Geometry check sheet. Reference: the model listing, model coordinates, mm. A direction names the side the tool comes from. Round coordinates to 2 decimals unless told otherwise and drop trailing zeros. Write each loop counter-clockwise with the first axis right and the second up, starting at its lowest first coordinate (ties: lowest second). Pieces come first, ordered by that corner, then holes.
Item 1: Draft check along Z on faces 6 (the face through (-20, -2, -20)), 7 (the face through (30, -1, 0)), 8 (the face through (32, -1, 0)), 9 (the face through (-12, -7, 5)). Enter one of: pulls with the +Z half, pulls with the -Z half, needs draft (parallel to the pull), parting line crosses it, or undercut.
Item 2: Access from +Z, -Z, +X, -X, +Y, -Y to the whole of each face (thin tool, end or side, straight path). Record for faces 1 (the face through (16.85, -22, 0)), 2 (the face through (-32, -1, 0)), 3 (the face through (22.5, -10, 0)), 4 (the face through (20, -2, -20)), 5 (the face through (-22.5, -34, 0)).
Item 3: Cross-section at A-A (z = -2). State how many separate pieces and enclosed holes the cut face has, then the cut area to 3 significant figures.
Item 4: Scan lines: probe 1 along X at (y, z) = (-25.5, 10); probe 2 along X at (y, z) = (-39, 8.5); probe 3 along Y at (x, z) = (-23, 10.5). Record each from-to range of solid material in increasing order.
Item 5: Cross-section at D-D (x = -11.5). Enter the section's corners in (y, z).
Item 6: Cross-section at B-B (y = -12.5). Enter the section's corners in (x, z).
Item 7: Depth check by flat-ended pin: P1, Ø17.5, axis at y = -30, z = -8, coming from the +X side; P2, Ø17.5, axis at y = -32, z = -4, coming from the -X side; P3, Ø4.5, axis at x = -18.5, z = -19.5, coming from the +Y side. Enter the tip coordinate at first touch or a pass-through.
Item 8: Cross-section at C-C (z = 18). Enter the section's corners in (x, y), then the cut area to 3 significant figures.
from build123d import *

# Parameters (mm, degrees)
F1_DEPTH      = 2
F2_W          = 5.6501800592
F2_H          = 10
F2_H_2        = 30
F3_DEPTH      = 40
F5_DEPTH      = 50
F7_DEPTH      = 50
F8_W          = 13.8498199408
F8_H          = 10
F9_DEPTH      = 15
F10_T4_DEPTH  = 87.150489639
F10_T10_DEPTH = 87.150489639


# Not quite as in the source:
# - a fillet or chamfer that OpenCascade refuses, or shapes differently, is made with other operations: its cross-section is extruded or revolved along the edge and cut away or added


with BuildPart() as f1:
    # F0 (on Front) → F1 (new body)
    with BuildSketch(Plane.XZ):
        with BuildLine():
            Line((32.5, 15), (-32.5, 15))
            ThreePointArc((-32.5, 15), (-34.267766953, 14.267766953), (-35, 12.5))
            Line((-35, 12.5), (-35, -12.5))
            ThreePointArc((-35, -12.5), (-34.267766953, -14.267766953), (-32.5, -15))
            Line((-32.5, -15), (32.5, -15))
            ThreePointArc((32.5, -15), (34.267766953, -14.267766953), (35, -12.5))
            Line((35, -12.5), (35, 12.5))
            ThreePointArc((35, 12.5), (34.267766953, 14.267766953), (32.5, 15))
        make_face()
        with BuildLine():
            Line((-32, -11), (-32, 11))
            ThreePointArc((-32, 11), (-31.7071067812, 11.7071067812), (-31, 12))
            ThreePointArc((-31, 12), (-30.2928932188, 11.7071067812), (-30, 11))
            Line((-30, 11), (-30, -11))
            ThreePointArc((-30, -11), (-30.2928932188, -11.7071067812), (-31, -12))
            ThreePointArc((-31, -12), (-31.7071067812, -11.7071067812), (-32, -11))
        make_face(mode=Mode.SUBTRACT)
        with BuildLine():
            Line((30, -11), (30, 11))
            ThreePointArc((30, 11), (30.2928932188, 11.7071067812), (31, 12))
            ThreePointArc((31, 12), (31.7071067812, 11.7071067812), (32, 11))
            Line((32, 11), (32, -11))
            ThreePointArc((32, -11), (31.7071067812, -11.7071067812), (31, -12))
            ThreePointArc((31, -12), (30.2928932188, -11.7071067812), (30, -11))
        make_face(mode=Mode.SUBTRACT)
    extrude(amount=F1_DEPTH)

    # F2 (on face) → F3 (join)
    with BuildSketch(Plane.XZ.offset(2)):
        with Locations((-19.6749099704, 20)):
            Rectangle(F2_W, F2_H)
        with Locations((-19.6749099704, 0)):
            Rectangle(F2_W, F2_H_2)
        with Locations((-19.6749099704, -20)):
            Rectangle(F2_W, F2_H)
        with Locations((19.6749099704, -20)):
            Rectangle(F2_W, F2_H)
        with Locations((19.6749099704, 0)):
            Rectangle(F2_W, F2_H_2)
        with Locations((19.6749099704, 20)):
            Rectangle(F2_W, F2_H)
    extrude(amount=F3_DEPTH)

    # F4 (on face) → F5 (cut, through all)
    with BuildSketch(Plane.XY.offset(25)):
        Polygon((-20.5, -17), (-22.5, -18), (-22.5, -26), (-20.5, -27), (-20.5, -26), (-20.5, -18), align=None)
    extrude(amount=-F5_DEPTH, mode=Mode.SUBTRACT)

    # F6 (on face) → F7 (cut, through all)
    with BuildSketch(Plane.XY.offset(25)):
        Polygon((22.5, -26), (22.5, -18), (20.5, -17), (20.5, -18), (20.5, -26), (20.5, -27), align=None)
    extrude(amount=-F7_DEPTH, mode=Mode.SUBTRACT)

    # F8 (on face) → F9 (join)
    with BuildSketch(Plane.XZ.offset(2)):
        with Locations((-9.9249099704, 0)):
            Rectangle(F8_W, F8_H)
        with Locations((9.9249099704, 0)):
            Rectangle(F8_W, F8_H)
    extrude(amount=F9_DEPTH)

    # F10: chamfer of 15 on 2 edges, made by hand


with BuildPart() as f10_tool2:
    # F10_s3 → F10_t4 (new body)
    with BuildSketch(Plane.XY.offset(-43.5752448195)):
        Polygon((-3, -2), (-18, -17), (-3, -17), align=None)
    extrude(amount=F10_T4_DEPTH)

    split(bisect_by=Plane.XZ.offset(2), keep=Keep.TOP)

    split(bisect_by=Plane.YZ.offset(-16.8498199408), keep=Keep.TOP)


with BuildPart() as f1_1:
    add(f1.part)

    # F10_t1: cut F10_tool2
    add(f10_tool2.part, mode=Mode.SUBTRACT)


with BuildPart() as f10_tool8:
    # F10_s9 → F10_t10 (new body)
    with BuildSketch(Plane.XY.offset(43.5752448195)):
        Polygon((3, -2), (18, -17), (3, -17), align=None)
    extrude(amount=-F10_T10_DEPTH)

    split(bisect_by=Plane.XZ.offset(2), keep=Keep.TOP)

    split(bisect_by=Plane.YZ.offset(16.8498199408), keep=Keep.BOTTOM)


with BuildPart() as f1_2:
    add(f1_1.part)

    # F10_t7: cut F10_tool8
    add(f10_tool8.part, mode=Mode.SUBTRACT)


solid = f1_2.part
Resolved:
1. face 6: needs draft
1. face 7: undercut
1. face 8: undercut
1. face 9: pulls with the +Z half
2. face 1: -Y
2. face 2: +Y, -Y
2. face 3: +Z, -Z, +X, -Y
2. face 4: -Z, +X, -X, +Y
2. face 5: +Z, -Z, -X, -Y
3. separate pieces: 3
3. enclosed holes: 0
3. area: 740 mm2
4. probe 1: x = -20.5 to -16.85, 16.85 to 20.5
4. probe 2: x = -22.5 to -16.85, 16.85 to 22.5
4. probe 3: y = -2 to 0
5. outline: (-10.5, -5) - (-2, -5) - (-2, -15) - (0, -15) - (0, 15) - (-2, 15) - (-2, 5) - (-10.5, 5) - close
6. outline: (-22.5, -25) - (-16.85, -25) - (-16.85, -5) - (-13.5, -5) - (-13.5, 5) - (-16.85, 5) - (-16.85, 25) - (-22.5, 25) - close; (13.5, -5) - (16.85, -5) - (16.85, -25) - (22.5, -25) - (22.5, 25) - (16.85, 25) - (16.85, 5) - (13.5, 5) - close
7. P1: stops at x = 22.5
7. P2: stops at x = -22.5
7. P3: stops at y = -2
8. outline: (-22.5, -42) - (-16.85, -42) - (-16.85, -2) - (-22.5, -2) - (-22.5, -18) - (-20.5, -17) - (-20.5, -27) - (-22.5, -26) - close; (16.85, -42) - (22.5, -42) - (22.5, -26) - (20.5, -27) - (20.5, -17) - (22.5, -18) - (22.5, -2) - (16.85, -2) - close
8. area: 416 mm2
